Read the model definition and answer for the solid it produces. Units are mm, in the model's axes. Face numbers are marked on the shaded views. Round coordinates to 2 decimals unless told otherwise and drop trailing zeros. Loops run counter-clockwise (first coordinate to the right, second up) from the corner with the lowest first, then second, coordinate; pieces in that order, holes last. Notation, with made-up numbers: (85, 61) -> (127, 61) arc R24 cw to (127, 99) -> close; hole circle Ø8 at (89, 12). An arc over 180 degrees is marked (long way). Put each result on its own line as item: value.
from build123d import *

# Parameters (mm, degrees)
SKETCH1_W           = 45
SKETCH1_H           = 20
SKETCH1_R           = 3
BOSS_EXTRUDE1_DEPTH = 3.1
SKETCH2_W           = 38.8
SKETCH2_H           = 5
BOSS_EXTRUDE2_DEPTH = 3.1


with BuildPart() as part:
    # Sketch1 → Boss-Extrude1 (new body)
    with BuildSketch(Plane.XY):
        Rectangle(SKETCH1_W, SKETCH1_H)
        Circle(SKETCH1_R, mode=Mode.SUBTRACT)
    extrude(amount=BOSS_EXTRUDE1_DEPTH)

    # Sketch2 → Boss-Extrude2 (add, through all)
    with BuildSketch(Plane.XY.offset(3.1)):
        with Locations((0, -12.5)):
            Rectangle(SKETCH2_W, SKETCH2_H)
    extrude(amount=-BOSS_EXTRUDE2_DEPTH)


solid = part.part
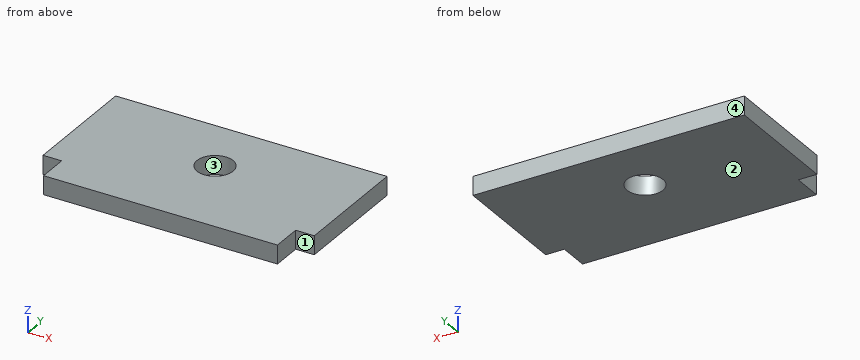
Item 1: The part is cut by section B-B (z = 2.5). Determine the outline of the cut face in (x, y).
Derived:
outline: (-22.5, -10) -> (-19.4, -10) -> (-19.4, -15) -> (19.4, -15) -> (19.4, -10) -> (22.5, -10) -> (22.5, 10) -> (-22.5, 10) -> close; hole circle Ø6 at (0, 0)
Item 2: The part is cut by section A-A (y = 0). Determine the outline of the cut face in (x, z), then the cut area to 3 significant figures.
Derived:
outline: (-22.5, 0) -> (-3, 0) -> (-3, 3.1) -> (-22.5, 3.1) -> close; (3, 0) -> (22.5, 0) -> (22.5, 3.1) -> (3, 3.1) -> close
area: 121 mm^2
Item 3: Flat-ended cylindrical pins translate along their axes: pin 1 Ø12 at (x, y) = (2, -3.5) entering from -Z; pin 2 Ø1.6 at (x, z) = (20.5, 1.5) entering from -Y. Find the tip coordinate at first contact, or state that the pin passes through.
Derived:
pin 1: stops at z = 0
pin 2: stops at y = -10
Item 4: The part is cut by section C-C (x = 0). Determine the outline of the cut face in (y, z), then the cut area to 3 significant figures.
Derived:
outline: (-15, 0) -> (-3, 0) -> (-3, 3.1) -> (-15, 3.1) -> close; (3, 0) -> (10, 0) -> (10, 3.1) -> (3, 3.1) -> close
area: 58.9 mm^2
Item 5: The part is cut by section D-D (y = -12.5). Determine the outline of the cut face in (x, z).
Derived:
outline: (-19.4, 0) -> (19.4, 0) -> (19.4, 3.1) -> (-19.4, 3.1) -> close
Item 6: Find the intervals of material crossed by line 1 along Y through (x, z) = (0, 0.85); line 2 along X through (y, z) = (-0.75, 0.5); line 3 along X through (y, z) = (-2.5, 2.55), in increasing order.
Derived:
line 1: y = -15 to -3, 3 to 10
line 2: x = -22.5 to -2.9, 2.9 to 22.5
line 3: x = -22.5 to -1.66, 1.66 to 22.5
Item 7: For a pull along Y with two mould halves and no side action, classify the marked faces 1, 2, 3 and 4 as pulls with the +Y half, pulls with the -Y half, needs draft (parallel to the pull), parting line crosses it, or undercut.
Derived:
face 1: pulls with the -Y half
face 2: needs draft
face 3: undercut
face 4: pulls with the +Y half
